```python
from build123d import *

# Parameters (mm, degrees)
BOSS_EXTRUDE1_DEPTH  = 4
M6_CLEARANCE_HOLE1_D = 7


with BuildPart() as part:
    # Sketch1 → Boss-Extrude1 (new body)
    with BuildSketch(Plane(origin=(0, 0, 0), x_dir=(1, 0, 0), z_dir=(0, 1, 0))):
        Polygon((0, 0), (-90, 0), (-90, 30), (-30, 90), (0, 90), align=None)
    extrude(amount=BOSS_EXTRUDE1_DEPTH)

    # M6 Clearance Hole1 (through all)
    with Locations(Plane(origin=(0, 4, 0), x_dir=(1, 0, 0), z_dir=(0, 1, 0))):
        with Locations((-75, 15), (-45, 15), (-15, 15), (-15, 45), (-15, 75)):
            Hole(M6_CLEARANCE_HOLE1_D / 2)


solid = part.part
```
CAD build for the part. Positions are in the model's coordinates, mm. Coordinates: 2 decimals unless noted, no trailing zeros. Write each loop counter-clockwise with the first axis right and the second up, starting at its lowest first coordinate (ties: lowest second). Pieces come first, ordered by that corner, then holes.
(1) Cut at D-D, the plane y = 1.6. List the corners of the cut face in (x, z), and give its area (3 significant figures).
(2) Two-plate mould, pull along X, no slides. Class faces 1 (the face through (-78.233, 1.972, -13.659)), 2 (the face through (-60, 2, -60)), 3 (the face through (-44, 2, 0)): +X half, -X half, draft (parallel to the pull), parting line (faces both ways), or undercut.
(3) Flat gauge pins, fed straight in: pin 1 (9 mm diameter, centred on x = -75, z = -15, fed in from -Y); pin 2 (1 mm diameter, centred on y = 0.5, z = -34.5, fed in from -X); pin 3 (6.5 mm diameter, centred on x = -15, z = -15, fed in from +Y). Where does each tip first touch, or does it go through?
(4) Cut at C-C, the plane x = -75. List the corners of the cut face in (y, z).
(5) Cut at A-A, the plane x = -15. List the corners of the cut face in (y, z).
(6) Drill centre lines: probe 1 along X at (y, z) = (3, -15); probe 2 along Z at (x, y) = (-45, 3.2). Where is each one in solid material? Low to high.
(7) Cut at B-B, the plane z = -75. List the corners of the cut face in (x, y).
Geometry says:
1. outline: (-90, -30) - (-30, -90) - (0, -90) - (0, 0) - (-90, 0) - close; hole circle Ø7 at (-75, -15); hole circle Ø7 at (-45, -15); hole circle Ø7 at (-15, -75); hole circle Ø7 at (-15, -45); hole circle Ø7 at (-15, -15)
1. area: 6,110 mm2
2. face 1: undercut
2. face 2: -X half
2. face 3: draft
3. pin 1: stops at y = 0
3. pin 2: stops at x = -86
3. pin 3: passes through
4. outline: (0, -45) - (4, -45) - (4, -18.5) - (0, -18.5) - close; (0, -11.5) - (4, -11.5) - (4, 0) - (0, 0) - close
5. outline: (0, -90) - (4, -90) - (4, -78.5) - (0, -78.5) - close; (0, -71.5) - (4, -71.5) - (4, -48.5) - (0, -48.5) - close; (0, -41.5) - (4, -41.5) - (4, -18.5) - (0, -18.5) - close; (0, -11.5) - (4, -11.5) - (4, 0) - (0, 0) - close
6. probe 1: x = -90 to -78.5, -71.5 to -48.5, -41.5 to -18.5, -11.5 to 0
6. probe 2: z = -75 to -18.5, -11.5 to 0
7. outline: (-45, 0) - (-18.5, 0) - (-18.5, 4) - (-45, 4) - close; (-11.5, 0) - (0, 0) - (0, 4) - (-11.5, 4) - close
